Autodesk Inventor part; units mm, degrees
ref_plane "YZ Plane" through (0, 0, 0) normal (1, 0, 0) x (0, 1, 0)
ref_plane "XZ Plane" through (0, 0, 0) normal (0, 1, 0) x (-1, 0, 0)
ref_plane "XY Plane" through (0, 0, 0) normal (0, 0, 1) x (1, 0, 0)
sketch "Sketch1" plane through (0, 0, 0) normal (0, 0, 1) x (1, 0, 0)
  line L0 (6.88, -5.08) -> (-6.88, -5.08)
  line L1 (-6.88, -5.08) -> (-6.88, 5.08)
  line L2 (-6.88, 5.08) -> (6.88, 5.08)
  line L3 (6.88, 5.08) -> (6.88, -5.08)
  line L4 (6.88, -5.08) -> (-6.88, 5.08) construction
  line L5 (-6.88, -5.08) -> (6.88, 5.08) construction
  circle A0 centre (0, 0) radius 3.6
  circle A1 centre (0, 0) radius 2.15
  line L6 (6.88, 0) -> (-6.88, 0)
  line L7 (0, 5.08) -> (0, -5.08)
  dimension "d0" = 13.76
  dimension "d1" = 10.16
  dimension "d2" = 7.2
  dimension "d3" = 4.3
extrude "Extrusion1" add sketch "Sketch1" along normal blind 9.379 contours L0 L7 A0 L6 L3 | L0 L1 L6 A0 L7 | L6 A0 L7 L2 L3 | L7 A1 L6 A0 | A0 L6 A1 L7 | L6 A1 L7 A0 | L1 L2 L7 A0 L6 | A0 L7 A1 L6
sketch "Sketch2" plane through (-6.88, 5.08, 0) normal (0, 1, 0) x (-1, 0, 0)
  line L0 (-12.08, 8.1) -> (-1.68, 8.1)
  line L1 (-6.88, 8.1) -> (-6.88, 9.379) construction
  line L2 (-13.76, 9.379) -> (0, 9.379) construction
  line L3 (-13.76, 9.379) -> (-12.76, 9.379)
  line L4 (0, 9.379) -> (-1, 9.379)
  line L5 (-12.08, 8.1) -> (-12.76, 9.379)
  line L6 (-1.68, 8.1) -> (-1, 9.379)
  line L7 (-13.76, 9.379) -> (-13.76, 11.379)
  line L8 (-13.76, 11.379) -> (0, 11.379)
  line L9 (0, 0) -> (0, 9.379) construction
  line L10 (0, 11.379) -> (0, 9.379)
  dimension "d6" = 10.4
  dimension "d19" = 1.279
  dimension "d20" = 1
  dimension "d21" = 1
  dimension "d22" = 2
extrude "Extrusion2" cut sketch "Sketch2" against normal up to next
properties part number "base_thorlabs"
For this review, take the finished solid that the model builds, in its own axes (mm). A direction names the side the tool comes from. Round coordinates to 2 decimals unless told otherwise and drop trailing zeros. Order: outer loops, then holes, each group sorted by start corner. A loop starts at its lowest first (then second) coordinate and runs counter-clockwise, first axis right, second up. Notation, with made-up numbers: (28, -16) -> (44, -16) arc R21 ccw to (44, -6) -> close; hole circle Ø10 at (76, 37). An arc over 180 degrees is marked (long way). Put each result on its own line as item: value.
Q1. Add section D-D on y = -4.5. Write out the cut boundary in (x, z), plus the area to 3 significant figures.
Check result:
outline: (-6.88, 0) -> (6.88, 0) -> (6.88, 9.38) -> (5.88, 9.38) -> (5.2, 8.1) -> (-5.2, 8.1) -> (-5.88, 9.38) -> (-6.88, 9.38) -> close
area: 115 mm2
Q2. Insertion check: pin 1 Ø2.5 at (x, y) = (0, 0) entering from -Z. The pin has a flat end and moves straight along its axis. Give the tip position at first contact, or say it passes through.
Check result:
pin 1: through
Q3. Add section C-C on z = 3. Write out the cut boundary in (x, y), plus the area to 3 significant figures.
Check result:
outline: (-6.88, -5.08) -> (6.88, -5.08) -> (6.88, 5.08) -> (-6.88, 5.08) -> close; hole circle Ø4.3 at (0, 0)
area: 125 mm2
Q4. Mouldability with a two-part tool opening along X and no side actions: class faces 3 (the flat face through (0, 5.08, 5)), 4 (the flat face through (-6.88, 0, 5)), 5 (the flat face through (5.535, 0.071, 8.731)) as pulls with the +X half, pulls with the -X half, needs draft (parallel to the pull), parting line crosses it, or undercut.
Check result:
face 3: needs draft
face 4: pulls with the -X half
face 5: undercut
Q5. For probe 1 along X at (y, z) = (0, 2.25); probe 2 along Y at (x, z) = (0, 5.5); probe 3 along Z at (x, y) = (-4.75, -2), list the stretches that pass through material, from the lowest coordinate up. Write a range as [from, to].
Check result:
probe 1: [-6.88, -2.15], [2.15, 6.88]
probe 2: [-5.08, -2.15], [2.15, 5.08]
probe 3: [0, 8.1]
Q6. Add section A-A on y = 0. Write out the cut boundary in (x, z), plus the area to 3 significant figures.
Check result:
outline: (-6.88, 0) -> (-2.15, 0) -> (-2.15, 8.1) -> (-5.2, 8.1) -> (-5.88, 9.38) -> (-6.88, 9.38) -> close; (2.15, 0) -> (6.88, 0) -> (6.88, 9.38) -> (5.88, 9.38) -> (5.2, 8.1) -> (2.15, 8.1) -> close
area: 80.1 mm2
Q7. Add section B-B on x = 0. Write out the cut boundary in (y, z).
Check result:
outline: (-5.08, 0) -> (-2.15, 0) -> (-2.15, 8.1) -> (-5.08, 8.1) -> close; (2.15, 0) -> (5.08, 0) -> (5.08, 8.1) -> (2.15, 8.1) -> close
Q8. Machinability: for faces 1 (the flat face through (6.4, 0.1, 9.379)), 2 (the flat face through (0.1, 2.3, 8.1)), which of the approach directions +Z, -Z, +X, -X, +Y, -Y give a long, thin tool a straight path to every point of the face, cutting with its end or side? Answer none if there is none.
Check result:
face 1: +Z, +X, -X, +Y, -Y
face 2: +Z, +Y, -Y
